Design review of the part built by this model. Coordinates are the model's own, in mm. Face numbers are marked on the shaded views. A direction names the side the tool comes from. Round coordinates to 2 decimals unless told otherwise and drop trailing zeros. Loops run counter-clockwise (first coordinate to the right, second up) from the corner with the lowest first, then second, coordinate; pieces in that order, holes last. Notation, with made-up numbers: M 65.5,87.5 L 84.5,87.5 A24 ccw 84.5,125.5 Z; hole C -22.75,-9 d7. An arc over 180 degrees is marked long. One line per item, written item: value. Start each with the question number.
Item 1: For the marked faces 1, 2, 3 and 4, list the 3-axis set-ups (+Z, -Z, +X, -X, +Y, -Y) from which the entire face can be reached by the end or side of a thin tool; tool diameter is ignored.
Item 2: We need section C-C (z = -1.25). Write out the cut boundary in (x, y) (3 decimals).
Item 3: For line 1 along Z through (x, y) = (-18.5, 11.75); line 2 along Z through (x, y) = (1.5, 0.5) (3 decimals); line 3 along X through (y, z) = (-0.75, 0) (3 decimals), list the stretches that pass through material, from the lowest coordinate up.
Item 4: We need section A-A (y = -4.5). Write out the cut boundary in (x, z) (3 decimals), then the cut area to 3 significant figures.
Item 5: Mouldability with a two-part tool opening along Z and no side actions: class the marked faces 5, 6, 7 and 8 as released by +Z, released by -Z, zero draft, split by the parting line, or undercut.
Item 6: We need section B-B (x = -20.5). Write out the cut boundary in (y, z) (3 decimals).
Item 7: Clearance check with flat-ended pins moving along their axes: pin 1 (2 mm diameter, centred on y = 6, z = -1.5, fed in from +X); pin 2 (3.5 mm diameter, centred on x = 11.5, z = -5, fed in from +Y); pin 3 (0.5 mm diameter, centred on x = -29, y = 8, fed in from -Z). State where each tip first meets the part, or that it passes through.
from build123d import *

# Parameters (mm, degrees)
EXTRUDE_1_DEPTH          = 2.25
EXTRUDE_2_DEPTH          = 12.61
FILLET_1_R               = 5
EXTRUDE_3_DEPTH          = 4.3
CUT_EXTRUDE_1_DEPTH      = 45.196553708
CUT_EXTRUDE_1_DEPTH_BACK = 15.68
SKETCH_4_W               = 53.83
SKETCH_4_H               = 4.15
SKETCH_4_W_2             = 1
SKETCH_4_H_2             = 7.5
SKETCH_4_W_3             = 1.585
SKETCH_4_H_3             = 5.4
SKETCH_4_W_4             = 2.705
SKETCH_4_W_5             = 1.12
SKETCH_4_H_4             = 2.17


with BuildPart() as part:
    # Эскиз1 → Бобышка-Вытянуть1 (new, symmetric)
    with BuildSketch(Plane(origin=(0, 0, 0), x_dir=(1, 0, 0), z_dir=(0, 1, 0))):
        with BuildLine():
            Line((-31.885, 11.595), (31.885, 11.595))
            ThreePointArc((31.885, 11.595), (35.420533906, 10.130533906), (36.885, 6.595))
            Line((36.885, 6.595), (36.885, -6.595))
            ThreePointArc((36.885, -6.595), (35.420533906, -10.130533906), (31.885, -11.595))
            Line((31.885, -11.595), (-31.885, -11.595))
            ThreePointArc((-31.885, -11.595), (-35.420533906, -10.130533906), (-36.885, -6.595))
            Line((-36.885, -6.595), (-36.885, 6.595))
            ThreePointArc((-36.885, 6.595), (-35.420533906, 10.130533906), (-31.885, 11.595))
        make_face()
    extrude(amount=EXTRUDE_1_DEPTH, both=True)

    # Эскиз2 → Бобышка-Вытянуть2 (add)
    with BuildSketch(Plane(origin=(0, 2.25, 0), x_dir=(1, 0, 0), z_dir=(0, 1, 0))):
        with BuildLine():
            ThreePointArc((-31.04, 5.32), (-31.038038076, 5.460054955), (-31.032153844, 5.6))
            Line((-31.032153844, 5.6), (-31.285, 5.6))
            ThreePointArc((-31.285, 5.6), (-36.885, 0), (-31.285, -5.6))
            Line((-31.285, -5.6), (-31.032153844, -5.6))
            ThreePointArc((-31.032153844, -5.6), (-31.038038076, -5.460054955), (-31.04, -5.32))
            Line((-31.04, -5.32), (-31.04, 5.32))
        make_face()
        with BuildLine():
            Line((31.032153844, -5.6), (-31.032153844, -5.6))
            ThreePointArc((-31.032153844, -5.6), (-29.475112807, -8.953180425), (-26.04, -10.32))
            Line((-26.04, -10.32), (26.04, -10.32))
            ThreePointArc((26.04, -10.32), (29.475112807, -8.953180425), (31.032153844, -5.6))
        make_face()
        with BuildLine():
            Line((31.032153844, 5.6), (-31.032153844, 5.6))
            ThreePointArc((-31.032153844, 5.6), (-31.038038076, 5.460054955), (-31.04, 5.32))
            Line((-31.04, 5.32), (-31.04, -5.32))
            ThreePointArc((-31.04, -5.32), (-31.038038076, -5.460054955), (-31.032153844, -5.6))
            Line((-31.032153844, -5.6), (31.032153844, -5.6))
            ThreePointArc((31.032153844, -5.6), (31.038038076, -5.460054955), (31.04, -5.32))
            Line((31.04, -5.32), (31.04, 5.32))
            ThreePointArc((31.04, 5.32), (31.038038076, 5.460054955), (31.032153844, 5.6))
        make_face()
        with BuildLine():
            Line((26.04, 10.32), (-26.04, 10.32))
            ThreePointArc((-26.04, 10.32), (-29.475112807, 8.953180425), (-31.032153844, 5.6))
            Line((-31.032153844, 5.6), (31.032153844, 5.6))
            ThreePointArc((31.032153844, 5.6), (29.475112807, 8.953180425), (26.04, 10.32))
        make_face()
        with BuildLine():
            Line((31.285, 5.6), (31.032153844, 5.6))
            ThreePointArc((31.032153844, 5.6), (31.038038076, 5.460054955), (31.04, 5.32))
            Line((31.04, 5.32), (31.04, -5.32))
            ThreePointArc((31.04, -5.32), (31.038038076, -5.460054955), (31.032153844, -5.6))
            Line((31.032153844, -5.6), (31.285, -5.6))
            ThreePointArc((31.285, -5.6), (36.885, 0), (31.285, 5.6))
        make_face()
    extrude(amount=EXTRUDE_2_DEPTH)

    # Скругление1
    fillet_1_edges = [part.edges().sort_by_distance(p)[0] for p in [
        (-31.032153844, 8.555, 5.6),
        (-31.032153844, 8.555, -5.6),
        (31.032153844, 8.555, -5.6),
        (31.032153844, 8.555, 5.6),
    ]]
    fillet(fillet_1_edges, radius=FILLET_1_R)

    # Эскиз3 → Бобышка-Вытянуть3 (add)
    with BuildSketch(Plane.XZ.offset(2.25)):
        with BuildLine():
            Line((-23.555, 10.465), (23.555, 10.465))
            ThreePointArc((23.555, 10.465), (27.090533906, 9.000533906), (28.555, 5.465))
            Line((28.555, 5.465), (28.555, -5.465))
            ThreePointArc((28.555, -5.465), (27.090533906, -9.000533906), (23.555, -10.465))
            Line((23.555, -10.465), (-23.555, -10.465))
            ThreePointArc((-23.555, -10.465), (-27.090533906, -9.000533906), (-28.555, -5.465))
            Line((-28.555, -5.465), (-28.555, 5.465))
            ThreePointArc((-28.555, 5.465), (-27.090533906, 9.000533906), (-23.555, 10.465))
        make_face()
    extrude(amount=EXTRUDE_3_DEPTH)

    # Эскиз4 → Вырез-Вытянуть1 (cut, two sides: drawn at the far end of the back side and taken through both)
    with BuildSketch(Plane(origin=(0, 14.86, 0), x_dir=(1, 0, 0), z_dir=(0, 1, 0)).offset(-CUT_EXTRUDE_1_DEPTH_BACK)):
        Polygon((26.915, 4.87), (-26.915, 4.87), (-26.915, -4.87), (26.915, -4.87), (26.915, -2.7), (25.795, -2.7), (25.795, 2.7), (26.915, 2.7), align=None)
        with Locations((0, 6.945)):
            Rectangle(SKETCH_4_W, SKETCH_4_H)
        with Locations((-29, 0)):
            Rectangle(SKETCH_4_W_2, SKETCH_4_H_2)
        with Locations((-28, 0)):
            Rectangle(SKETCH_4_W_2, SKETCH_4_H_2)
        Polygon((-26.915, -4.87), (-26.915, 4.87), (-28.5, 4.87), (-28.5, 3.75), (-27.5, 3.75), (-27.5, -3.75), (-28.5, -3.75), (-28.5, -4.87), align=None)
        with Locations((0, -6.945)):
            Rectangle(SKETCH_4_W, SKETCH_4_H)
        with Locations((27.7075, 0)):
            Rectangle(SKETCH_4_W_3, SKETCH_4_H_3)
        with Locations((29.8525, 0)):
            Rectangle(SKETCH_4_W_4, SKETCH_4_H_3)
        with Locations((26.355, 0)):
            Rectangle(SKETCH_4_W_5, SKETCH_4_H_3)
        with Locations((27.7075, -3.785)):
            Rectangle(SKETCH_4_W_3, SKETCH_4_H_4)
        with Locations((27.7075, 3.785)):
            Rectangle(SKETCH_4_W_3, SKETCH_4_H_4)
    extrude(amount=CUT_EXTRUDE_1_DEPTH + CUT_EXTRUDE_1_DEPTH_BACK, mode=Mode.SUBTRACT)


solid = part.part
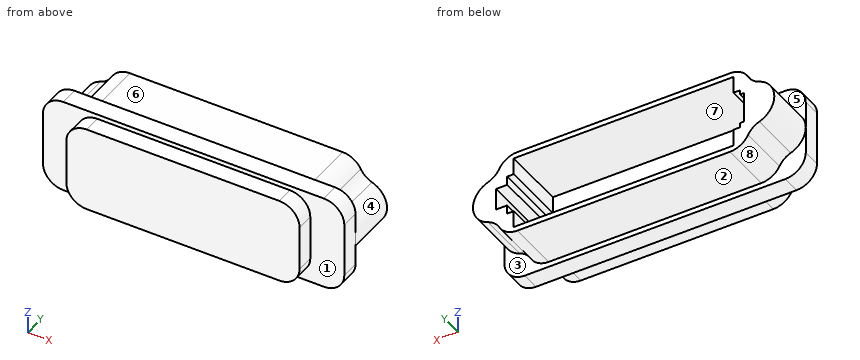
A:
1. face 1: -Y
1. face 2: -Z, +X, -X, +Y
1. face 3: -Z, +Y
1. face 4: +X, +Y
2. outline: M -36.885,-2.25 L -28.555,-2.25 L -28.555,-6.55 L 28.555,-6.55 L 28.555,-2.25 L 36.885,-2.25 L 36.885,2.25 L 36.744,2.25 L 36.744,14.86 L 31.205,14.86 L 31.205,-0.82 L -29.5,-0.82 L -29.5,14.86 L -36.744,14.86 L -36.744,2.25 L -36.885,2.25 Z
3. line 1: -10.32 to -9.02, 9.02 to 10.32
3. line 2: -11.595 to -9.02, 9.02 to 11.595
3. line 3: -36.885 to -29.5, 31.205 to 36.885
4. outline: M -28.555,-5.465 A5 ccw -23.555,-10.465 L 23.555,-10.465 A5 ccw 28.555,-5.465 L 28.555,5.465 A5 ccw 23.555,10.465 L -23.555,10.465 A5 ccw -28.555,5.465 Z
4. area: 1,170 mm2
5. face 5: zero draft
5. face 6: released by +Z
5. face 7: undercut
5. face 8: released by -Z
6. outline: M -6.55,-10.465 L -2.25,-10.465 L -2.25,-11.595 L 2.25,-11.595 L 2.25,-10.32 L 14.86,-10.32 L 14.86,-9.02 L -0.82,-9.02 L -0.82,9.02 L 14.86,9.02 L 14.86,10.32 L 2.25,10.32 L 2.25,11.595 L -2.25,11.595 L -2.25,10.465 L -6.55,10.465 Z
7. pin 1: x = 36.86
7. pin 2: y = -0.82
7. pin 3: z = -9.52
